Check sheet for the modelled part. Datum: model origin and axes. Units: mm. Give positions to 0.01 mm unless a question says otherwise; leave off trailing zeros. Write each loop counter-clockwise with the first axis right and the second up, starting at its lowest first coordinate (ties: lowest second). Pieces come first, ordered by that corner, then holes. Notation, with made-up numbers: (60.25, 83.5) -> (95.25, 83.5) arc R31 cw to (95.25, 113.5) -> close; hole circle Ø1 at (29.25, 56.5). An arc over 180 degrees is marked (long way). Answer as a JSON object with one key per item and string values.
from build123d import *

# Parameters (mm, degrees)
SKETCH1_R           = 2.38125
BOSS_EXTRUDE1_DEPTH = 10
FILLET5_R           = 3
FILLET6_R           = 1
FILLET7_R           = 2


with BuildPart() as part:
    # Sketch1 → Boss-Extrude1 (new body)
    with BuildSketch(Plane.XY):
        with BuildLine():
            Line((12.5, -4), (0.5, 8))
            Line((0.5, 8), (-12.5, 8))
            Line((-12.5, 8), (-12.5, 3))
            ThreePointArc((-12.5, 3), (-11.31971292, -0.189443986), (-12.098076211, -3.5))
            ThreePointArc((-12.098076211, -3.5), (-12.397777479, -4.223542865), (-12.5, -5))
            ThreePointArc((-12.5, -5), (-11.621320344, -7.121320344), (-9.5, -8))
            Line((-9.5, -8), (12.5, -8))
            Line((12.5, -8), (12.5, -4))
        make_face()
        with Locations((-9, 4.5)):
            Circle(SKETCH1_R, mode=Mode.SUBTRACT)
    extrude(amount=BOSS_EXTRUDE1_DEPTH)

    # Fillet5
    fillet5_edges = [part.edges().sort_by_distance(p)[0] for p in [
        (0.5, 8, 5),
    ]]
    fillet(fillet5_edges, radius=FILLET5_R)

    # Fillet6
    fillet6_edges = [part.edges().sort_by_distance(p)[0] for p in [
        (12.5, -8, 5),
    ]]
    fillet(fillet6_edges, radius=FILLET6_R)

    # Fillet7
    fillet7_edges = [part.edges().sort_by_distance(p)[0] for p in [
        (-12.5, 8, 5),
    ]]
    fillet(fillet7_edges, radius=FILLET7_R)


solid = part.part
1. Sectioned sample at D-D, the plane x = 3.75. Enter the section's corners in (y, z).
Determined:
{"outline": "(-8, 0) -> (4.75, 0) -> (4.75, 10) -> (-8, 10) -> close"}
2. Sectioned sample at C-C, the plane z = 7.75. Enter the section's corners in (x, y), plus the area to 3 significant figures.
Determined:
{"outline": "(-12.5, 3) arc R5.89 cw to (-12.1, -3.5) arc R3 ccw to (-9.5, -8) -> (11.5, -8) arc R1 ccw to (12.5, -7) -> (12.5, -4) -> (1.38, 7.12) arc R3 ccw to (-0.74, 8) -> (-10.5, 8) arc R2 ccw to (-12.5, 6) -> close; hole circle Ø4.76 at (-9, 4.5)", "area": "301 mm^2"}
3. Scan lines: L1, parallel to Y at x = -9, z = 4.25; L2, parallel to X at y = -1.5, z = 5; L3, parallel to X at y = 6.5, z = 6.25. Record each from-to range of solid material in increasing order. Write a range as [from, to].
Determined:
{"L1": "[-8, 2.12], [6.88, 8]", "L2": "[-11.39, 10]", "L3": "[-12.44, -10.29], [-7.71, 2]"}
4. Go/stop test with flat-tipped pins: P1, Ø6, axis at y = 2, z = 5.5, coming from the -X side; P2, Ø4, axis at y = 4, z = 2, coming from the +X side. Record where each tip stops, or that it passes through.
Determined:
{"P1": "x = -12.5", "P2": "x = 6.5"}
5. Sectioned sample at A-A, the plane y = 4.5. Enter the section's corners in (x, z).
Determined:
{"outline": "(-12.5, 0) -> (-11.38, 0) -> (-11.38, 10) -> (-12.5, 10) -> close; (-6.62, 0) -> (4, 0) -> (4, 10) -> (-6.62, 10) -> close"}
6. Sectioned sample at B-B, the plane x = -9. Enter the section's corners in (y, z).
Determined:
{"outline": "(-8, 0) -> (2.12, 0) -> (2.12, 10) -> (-8, 10) -> close; (6.88, 0) -> (8, 0) -> (8, 10) -> (6.88, 10) -> close"}
7. Mould release check, pull along Y, two halves, no side actions. Record for faces 1 (the face through (-3, -2, 0)), 2 (the face through (-11.323, -0.141, 4.93)), 3 (the face through (12.215, -7.699, 5.07)): released by +Y, released by -Y, zero draft, split by the parting line, or undercut.
Determined:
{"face 1": "zero draft", "face 2": "undercut", "face 3": "released by -Y"}
